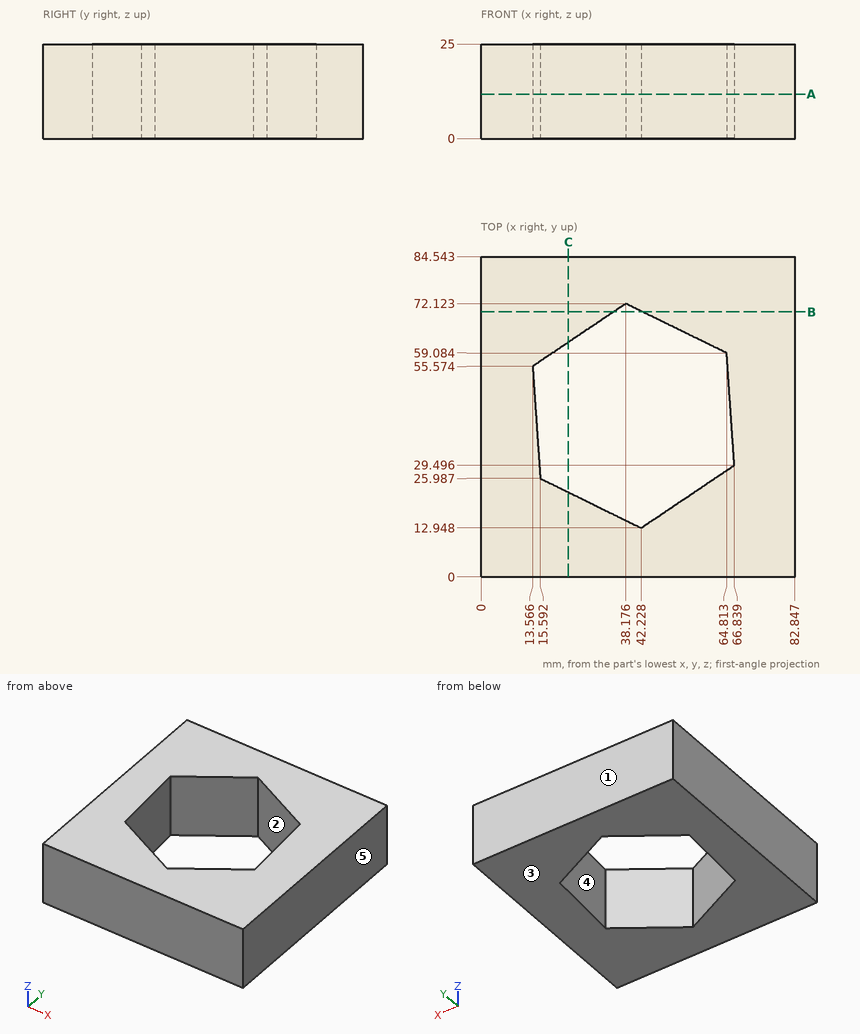
Answer from the drawing. Dimensions are ordinates in mm from the lowest x, y and z of the part. A direction names the side the tool comes from. Coordinates: 2 decimals unless noted, no trailing zeros. Write each loop counter-clockwise with the first axis right and the second up, starting at its lowest first coordinate (ties: lowest second). Pieces come first, ordered by that corner, then holes. Notation, with made-up numbers: M 33.5,25 L 54.5,25 A22 ccw 54.5,51 Z; hole C 30,-26 d10. An arc over 180 degrees is marked long. Use one line per item in the form item = value. Start each with the question number.
1. The part is cut by section B-B (y = 70). Give the vertices of the cut face in (x, z), plus the area to 3 significant figures.
2. The part is cut by section A-A (z = 11.75). Give the vertices of the cut face in (x, y) (1 decimal), plus the area to 3 significant figures.
3. The part is cut by section C-C (x = 23). Give the vertices of the cut face in (y, z).
4. A tool of negligible diameter and unlimited length cuts with its end or side. For the marked faces 1 and 2, from which of +Z, -Z, +X, -X, +Y, -Y can it reach the whole face along a straight path? Write none if from no direction.
5. Straight lines are drawn through the part: probe 1 along X at (y, z) = (33, 12.5); probe 2 along Y at (x, z) = (18, 15.75) (1 decimal); probe 3 along Y at (x, z) = (27.5, 22.5) (1 decimal). For each, find the intervals that lie inside material, in ascending order. Write a range as from..to.
6. The mould has two halves that part along X. Classify the marked faces 3, 4 and 5: released by +X, released by -X, zero draft, split by the parting line, or undercut.
Evaluation:
q1.outline = M 0,0 L 35.02,0 L 35.02,25 L 0,25 Z; M 42.51,0 L 82.85,0 L 82.85,25 L 42.51,25 Z
q1.area = 1,880 mm^2
q2.outline = M 0,0 L 82.8,0 L 82.8,84.5 L 0,84.5 Z; hole M 13.6,55.6 L 15.6,26 L 42.2,12.9 L 66.8,29.5 L 64.8,59.1 L 38.2,72.1 Z
q2.area = 4,720 mm^2
q3.outline = M 0,0 L 22.36,0 L 22.36,25 L 0,25 Z; M 61.92,0 L 84.54,0 L 84.54,25 L 61.92,25 Z
q4.face_1 = +Z, -Z, +X, -X, +Y
q4.face_2 = +Z, -Z
q5.probe_1 = 0..15.11, 66.6..82.85
q5.probe_2 = 0..24.8, 58.6..84.5
q5.probe_3 = 0..20.2, 64.9..84.5
q6.face_3 = zero draft
q6.face_4 = undercut
q6.face_5 = released by +X
